Design review of the part built by this model. Coordinates are the model's own, in mm. A direction names the side the tool comes from. Round coordinates to 2 decimals unless told otherwise and drop trailing zeros. Order: outer loops, then holes, each group sorted by start corner. A loop starts at its lowest first (then second) coordinate and runs counter-clockwise, first axis right, second up. Notation, with made-up numbers: (-2, -7) - (14, -7) arc R26 cw to (14, 19) - close; hole circle Ø11 at (82.25, 56.5). An arc over 180 degrees is marked (long way). Use CSV: the item, a comma, the result in double quotes. Start each with the question number.
from build123d import *

# Parameters (mm, degrees)
SKETCH_R     = 4
PAD_DEPTH    = 6
SKETCH001_R  = 1.4
PAD001_DEPTH = 2
CHAMFER_SIZE = 1.99
SKETCH002_R  = 1.05
POCKET_DEPTH = 4


with BuildPart() as part:
    # Sketch → Pad (new body)
    with BuildSketch(Plane.XY):
        Circle(SKETCH_R)
    extrude(amount=PAD_DEPTH)

    # Sketch001 (on Face3 of Pad) → Pad001 (join)
    with BuildSketch(Plane.XY.offset(6)):
        Circle(SKETCH001_R)
    extrude(amount=PAD001_DEPTH)

    # Chamfer
    chamfer_edges = [part.edges().sort_by_distance(p)[0] for p in [
        (-1.4, 0, 6),
    ]]
    chamfer(chamfer_edges, length=CHAMFER_SIZE)

    # Sketch002 (on Face6 of Chamfer) → Pocket (cut)
    with BuildSketch(Plane.XY.offset(8)):
        Circle(SKETCH002_R)
    extrude(amount=-POCKET_DEPTH, mode=Mode.SUBTRACT)


solid = part.part
Q1. The part is to be moulded in two halves that separate along Y. For faces 1 (the cylindrical face through (-0.867, -3.905, 2.958)), 2 (the flat face through (-3, 2, 6)), 3 (the flat face through (0, 0, 4)), say which applies: +Y half, -Y half, draft (parallel to the pull), parting line (faces both ways), or undercut.
Q2. Take a section at B-B (z = 4.5). State the section outline as (x, y) points.
Q3. Clearance check with flat-ended pins moving along their axes: pin 1 (1.5 mm diameter, centred on x = 1.5, y = -2.5, fed in from +Z); pin 2 (1.9 mm diameter, centred on x = 0, y = 0, fed in from +Z); pin 3 (4 mm diameter, centred on y = -3, z = 1, fed in from +X). State where each tip first meets the part, or that it passes through.
Q4. Tool access review of faces 4 (the cylindrical face through (1, 0.32, 6.03)), 5 (the flat face through (0, 0, 0)): name each direction out of +Z, -Z, +X, -X, +Y, -Y from which nothing blocks a thin tool from reaching the whole face with its end or side.
Q5. For L1, parallel to Y at x = 0, z = 5.4; L2, parallel to Y at x = 0, z = 6.5; L3, parallel to Z at x = 3, y = -2.5, list the stretches that pass through material, from the lowest coordinate up. Write a range as [from, to].
Q6. Take a section at D-D (z = 2.5). State the section outline as (x, y) points, plus the area to 3 significant figures.
Findings below:
1,face 1,"parting line"
1,face 2,"draft"
1,face 3,"undercut"
2,outline,"circle Ø8 at (0, 0); hole circle Ø2.1 at (0, 0)"
3,pin 1,"stops at z = 7.22"
3,pin 2,"stops at z = 4"
3,pin 3,"stops at x = 3.87"
4,face 4,"+Z"
4,face 5,"-Z, +X, -X, +Y, -Y"
5,L1,"y = [-4, -1.05], [1.05, 4]"
5,L2,"y = [-2.89, -1.05], [1.05, 2.89]"
5,L3,"z = [0, 6]"
6,outline,"circle Ø8 at (0, 0)"
6,area,"50.3 mm^2"
